Source: CAD feature listing. Evaluate the final solid. Frame: model axes, mm. Face numbers are marked on the shaded views. A direction names the side the tool comes from. Coordinates: 2 decimals unless noted, no trailing zeros. Order: outer loops, then holes, each group sorted by start corner. A loop starts at its lowest first (then second) coordinate and runs counter-clockwise, first axis right, second up.
Item 1: Section C-C on z = 0. Return the cut outline in (x, y), then the cut area to 3 significant figures.
Item 2: Ray query, line 1 (Z direction, x = 0, y = -144); line 2 (X direction, y = -53, z = -52.5) (3 decimals); line 3 (Z direction, x = -7.5, y = -249). Return the intervals inside material, ascending.
Item 3: Section B-B on x = 0. Return the cut outline in (y, z), then the cut area to 3 significant figures.
Item 4: Reachability of the marked faces 1 and 2 from +Z, -Z, +X, -X, +Y, -Y: full face, straight path, thin tool, end or side. Return the list, or none.
Item 5: Section A-A on y = -223. Return the cut outline in (x, z) (3 decimals), then the cut area to 3 significant figures.
Item 6: Contact query for flat-ended pins moving along their axis: P1, Ø10, axis at x = 0, y = -210.5, coming from the -Z side; P2, Ø11.5, axis at x = 0, z = 0, coming from the -Y side; P3, Ø3, axis at y = -211, z = -11, coming from the +X side; P4, Ø8, axis at y = -36, z = 4, coming from the +X side. Output: stop coordinate, or through.
Item 7: Section D-D on z = -32.5. Return the cut outline in (x, y) (3 decimals).
from build123d import *

# Parameters (mm, degrees)
F0_R     = 6.35
F1_DEPTH = 304.8


# Not quite as in the source:
# - a feature names something its author has since deleted; it is built from what else it names


with BuildPart() as f1:
    # F0 (on Front) → F1 (new body)
    with BuildSketch(Plane.XZ):
        Polygon((-9.525, -12.7128391741), (-12.7, -12.7), (-12.7, -57.5586806671), (-9.525, -57.5586806671), align=None)
        Polygon((15.8747663651, -12.8155516218), (13.7463785204, 12.7), (-12.7, 12.7), (-12.7, -12.7), (-9.525, -12.7), (-9.525, -12.7128391741), align=None)
        Circle(F0_R, mode=Mode.SUBTRACT)
        Polygon((-9.525, -12.7), (-12.7, -12.7), (-9.525, -12.7128391741), align=None)
    extrude(amount=F1_DEPTH)


solid = f1.part
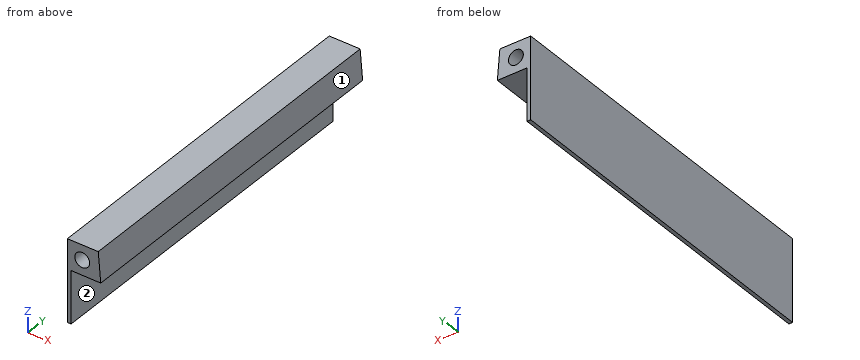
Answer list:
1. outline: (-12.7, -304.8) - (-6.35, -304.8) - (-6.35, 0) - (-12.7, 0) - close; (6.35, -304.8) - (14.81, -304.8) - (14.81, 0) - (6.35, 0) - close
1. area: 4,510 mm2
2. line 1: z = -12.75 to -6.35, 6.35 to 12.7
2. line 2: x = -12.7 to -9.525
2. line 3: z = -12.72 to 12.7
3. outline: (-304.8, -12.75) - (0, -12.75) - (0, -6.35) - (-304.8, -6.35) - close; (-304.8, 6.35) - (0, 6.35) - (0, 12.7) - (-304.8, 12.7) - close
3. area: 3,890 mm2
4. face 1: +Z, +X, +Y, -Y
4. face 2: -Z, +X, +Y, -Y
5. outline: (-12.7, -57.559) - (-9.525, -57.559) - (-9.525, -12.713) - (15.875, -12.816) - (13.746, 12.7) - (-12.7, 12.7) - close; hole circle Ø12.7 at (0, 0)
5. area: 716 mm2
6. P1: stops at z = -12.77
6. P2: passes through
6. P3: stops at x = 15.85
6. P4: stops at x = 14.81
7. outline: (-12.7, -304.8) - (-9.525, -304.8) - (-9.525, 0) - (-12.7, 0) - close
